```python
from build123d import *

# Parameters (mm, degrees)
F0_R      = 53.5
F1_DEPTH  = 13
F2_T      = -3
F3_R      = 48
F3_R_2    = 42.25
F3_R_3    = 37
F4_DEPTH  = 2.5
F5_DEPTH  = 8
F6_SIZE2  = 6
F6_SIZE   = 3
F7_SIZE2  = 1.5
F7_SIZE   = 4
F8_R      = 1
F9_R      = 5
F10_DEPTH = 45.7
F11_W     = 50.4
F11_H     = 50.4
F12_DEPTH = 1.5


with BuildPart() as f1:
    # F0 (on Top) → F1 (new body)
    with BuildSketch(Plane.XY):
        Circle(F0_R)
    extrude(amount=F1_DEPTH)

    # F2
    f2_openings = [f1.faces().sort_by_distance(p)[0] for p in [
        (0, 0, 13),
    ]]
    offset(amount=F2_T, openings=f2_openings)

    # F3 (on face) → F4 (join)
    with BuildSketch(Plane.XY.offset(3)):
        Circle(F3_R)
        Circle(F3_R_2, mode=Mode.SUBTRACT)
        Circle(F3_R_2)
        Circle(F3_R_3, mode=Mode.SUBTRACT)
    extrude(amount=F4_DEPTH)

    # F3 (on face) → F5 (join)
    with BuildSketch(Plane.XY.offset(3)):
        Circle(F3_R_2)
        Circle(F3_R_3, mode=Mode.SUBTRACT)
    extrude(amount=F5_DEPTH)

    # F6
    f6_edges = [f1.edges().sort_by_distance(p)[0] for p in [
        (-37, 0, 11),
    ]]
    f6_side = f1.faces().sort_by_distance((-41.05499, 0, 11))[0]
    chamfer(f6_edges, length=F6_SIZE, length2=F6_SIZE2, reference=f6_side)

    # F7
    f7_edges = [f1.edges().sort_by_distance(p)[0] for p in [
        (-50.5, 0, 13),
    ]]
    chamfer(f7_edges, length=F7_SIZE, length2=F7_SIZE2)

    # F8
    f8_edges = [f1.edges().sort_by_distance(p)[0] for p in [
        (-48, 0, 5.5),
        (-53.5, 0, 0),
        (-53.5, 0, 13),
    ]]
    fillet(f8_edges, radius=F8_R)

    # F9 (on face) → F10 (cut, symmetric)
    with BuildSketch(Plane.XY.offset(5.5)):
        Circle(F9_R)
    extrude(amount=F10_DEPTH, both=True, mode=Mode.SUBTRACT)

    # F11 (on face) → F12 (cut)
    with BuildSketch(Plane.XY.offset(3)):
        Rectangle(F11_W, F11_H)
    extrude(amount=-F12_DEPTH, mode=Mode.SUBTRACT)


solid = f1.part
```
Check sheet for the modelled part. Datum: model origin and axes. Units: mm. A direction names the side the tool comes from. Give positions to 0.01 mm unless a question says otherwise; leave off trailing zeros. One line per question, with ' | ' between items. Start each with the question number.
1. Gauge pin test, flat ends, axial feed: pin 1 Ø0.8 at (x, z) = (-8.5, 2) entering from +Y; pin 2 Ø1 at (x, z) = (-17, 11.5) entering from -Y; pin 3 Ø2 at (y, z) = (-30, 9) entering from -X; pin 4 Ø13 at (x, y) = (0, 0) entering from -Z. Record the tip position at first contact, or that the pin passes through.
2. Material ranges on line 1 along Y through (x, z) = (0, 4.5); line 2 along Y through (x, z) = (21, 7.25); line 3 along X through (y, z) = (29, 6.75), recorded low to high. Write a range as [from, to].
3. Draft check along Y on faces 1 (the cylindrical face through (-31.1, 28.6, 8.2)), 2 (the flat face through (-1, -11, 0)), 3 (the cylindrical face through (-11.598, -52.228, 6.423)). Enter one of: released by +Y, released by -Y, zero draft, split by the parting line, or undercut.
4. Set-up check for faces 4 (the flat face through (37.4, -15.5, 11)), 5 (the cylindrical face through (-1.08, -4.88, 0.76)): record each of +Z, -Z, +X, -X, +Y, -Y from which the full face is reachable in a straight line by a thin tool's end or side.
Check result:
1) pin 1: stops at y = 52.88 | pin 2: stops at y = -50.89 | pin 3: stops at x = -44.96 | pin 4: stops at z = 0
2) line 1: y = [-53.5, -50.5], [-48, -37], [37, 48], [50.5, 53.5] | line 2: y = [-49.21, -45.93], [-36.66, -31.82], [31.82, 36.66], [45.93, 49.21] | line 3: x = [-44.96, -41.34], [-30.73, -24.36], [24.36, 30.73], [41.34, 44.96]
3) face 1: undercut | face 2: zero draft | face 3: split by the parting line
4) face 4: +Z | face 5: +Z, -Z
